Answer from the drawing. Dimensions are ordinates in mm from the lowest x, y and z of the part. A direction names the side the tool comes from. Give positions to 0.01 mm unless a question says otherwise; leave off trailing zeros. Write each loop counter-clockwise with the first axis right and the second up, starting at its lowest first coordinate (ties: lowest second). Pieces come first, ordered by that corner, then holes. Notation, with made-up numbers: M 79,-36 L 107,-36 A23 cw 107,-13 Z; hole C 57,49 d3. An arc over 180 degrees is marked long. Put each result on its own line as item: value.
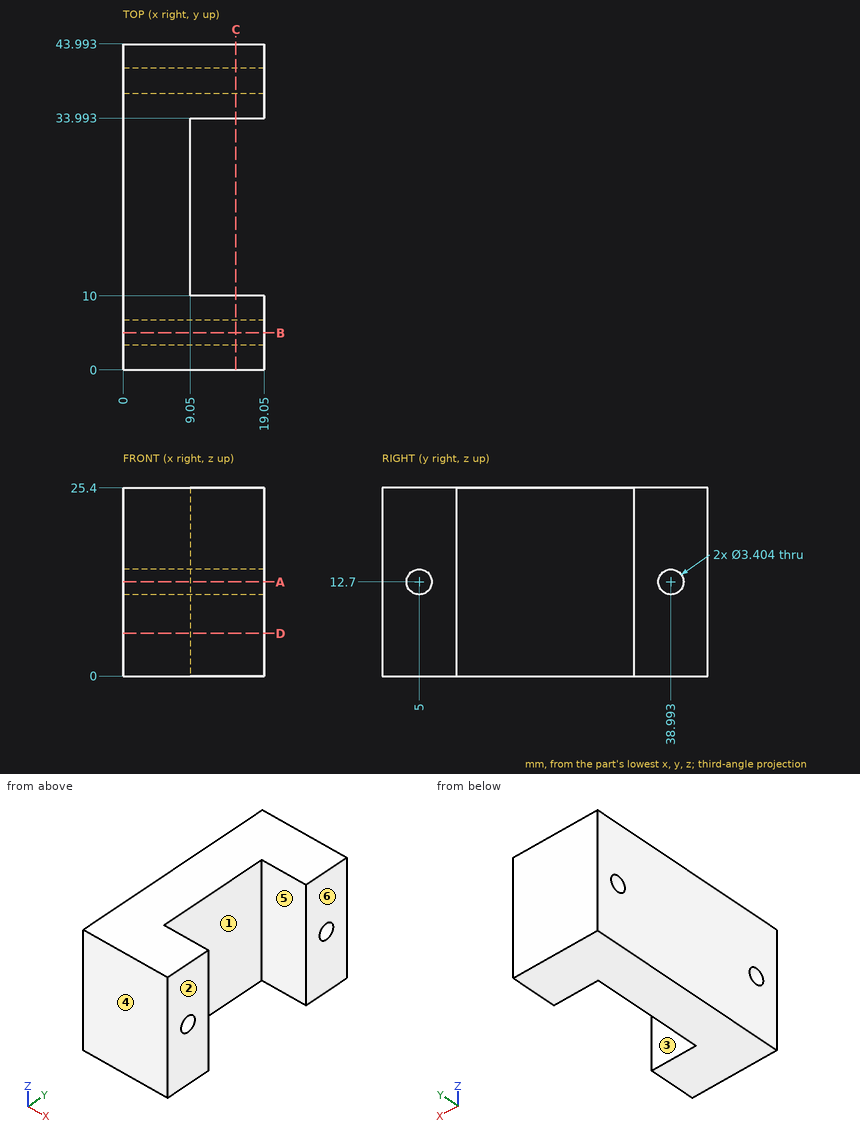
(1) For a pull along Y with two mould halves and no side action, classify the marked faces 3, 4, 5 and 6 as +Y half, -Y half, draft (parallel to the pull), parting line (faces both ways), or undercut.
Result:
face 3: undercut
face 4: -Y half
face 5: undercut
face 6: draft
(2) Straight lines are drawn through the part: line 1 along Y through (x, z) = (7.25, 12.7) (1 decimal); line 2 along Y through (x, z) = (12.75, 12.7) (1 decimal); line 3 along Y through (x, z) = (11, 16). For each, find the intervals that lie inside material, in ascending order. Write a range as from..to.
Result:
line 1: y = 0..3.3, 6.7..37.3, 40.7..44
line 2: y = 0..3.3, 6.7..10, 34..37.3, 40.7..44
line 3: y = 0..10, 33.99..43.99
(3) Which of the six approach directions +Z, -Z, +X, -X, +Y, -Y give full straight-line access (tool end or side, diameter ignored) to the marked faces 1 and 2?
Result:
face 1: +Z, -Z, +X
face 2: +Z, -Z, +X, +Y, -Y
(4) Given pin 1 Ø2.5 at (y, z) = (5, 12.7) entering from +X; pin 2 Ø12 at (y, z) = (21.5, 15) entering from +X, each flat-ended and moving along its own axis, determine where each tip first touches the part or whether it passes through.
Result:
pin 1: passes through
pin 2: stops at x = 9.05
(5) Section B-B on y = 5 is taken. Determine the outline of the cut face in (x, z), and give its area (3 significant figures).
Result:
outline: M 0,0 L 19.05,0 L 19.05,11 L 0,11 Z; M 0,14.4 L 19.05,14.4 L 19.05,25.4 L 0,25.4 Z
area: 419 mm²
(6) Section C-C on x = 15.25 is taken. Determine the outline of the cut face in (y, z), and give its area (3 significant figures).
Result:
outline: M 0,0 L 10,0 L 10,25.4 L 0,25.4 Z; M 33.99,0 L 43.99,0 L 43.99,25.4 L 33.99,25.4 Z; hole C 5,12.7 d3.4; hole C 38.99,12.7 d3.4
area: 490 mm²
(7) Section A-A on z = 12.7 is taken. Give the number of separate pieces and of enclosed holes in the cut face.
Result:
separate pieces: 3
enclosed holes: 0
(8) Section D-D on z = 5.75 is taken. Determine the outline of the cut face in (x, y).
Result:
outline: M 0,0 L 19.05,0 L 19.05,10 L 9.05,10 L 9.05,33.99 L 19.05,33.99 L 19.05,43.99 L 0,43.99 Z
